The model under review builds one solid part; all positions refer to its coordinate system, in mm. A direction names the side the tool comes from. Round coordinates to 2 decimals unless told otherwise and drop trailing zeros. Order: outer loops, then holes, each group sorted by start corner. A loop starts at its lowest first (then second) coordinate and runs counter-clockwise, first axis right, second up. Notation, with made-up numbers: M 20,-13 L 30,-13 A16 cw 30,-9 Z; hole C 58.25,-1.75 d5. An arc over 180 degrees is marked long. Answer as a JSON object with one key per item and string values. Group by question number.
1) The part is to be moulded in two halves that separate along X. For faces 1 (the flat face through (-17, 16, -24)), 2 (the conical face through (-9.1, 9, 18.8)), 3 (the flat face through (-24, 0, 0)), say which applies: +X half, -X half, draft (parallel to the pull), parting line (faces both ways), or undercut.
2) For faces 4 (the flat face through (-17, 16, 24)), 5 (the conical face through (9.1, -9, 18.8)), list the 3-axis set-ups (+Z, -Z, +X, -X, +Y, -Y) from which the entire face can be reached by the end or side of a thin tool; tool diameter is ignored.
3) To check wall thickness, follow line 1 (X direction, y = 0, z = 4.5); line 2 (Y direction, x = -0.5, z = 5.5); line 3 (X direction, y = -2, z = 8). State the ranges of each line that lie inside material, in increasing order.
4) Insertion check: pin 1 Ø6 at (x, y) = (-17, 0) entering from +Z. The pin has a flat end and moves straight along its axis. Give the tip position at first contact, or say it passes through.
5) Consider section B-B, the plane x = -17. Write out the cut boundary in (y, z), then the cut area to 3 significant figures.
6) Consider section A-A, the plane z = -10. Write out the cut boundary in (x, y), then the cut area to 3 significant figures.
```python
from build123d import *

# Parameters (mm, degrees)
F0_W           = 48
F0_H           = 48
F1_DEPTH       = 24
F2_R           = 9
F3_DEPTH       = 48
F6_D           = 18
F6_CSINK_D     = 36
F6_CSINK_ANGLE = 90
F4_R           = 9
F7_DEPTH       = 48


with BuildPart() as f1:
    # F0 (on Front) → F1 (new body, symmetric)
    with BuildSketch(Plane.XZ):
        Rectangle(F0_W, F0_H)
    extrude(amount=F1_DEPTH, both=True)

    # F2 (on face) → F3 (cut)
    with BuildSketch(Plane.XZ.offset(24)):
        with Locations((0, 24)):
            Circle(F2_R)
        with Locations((0, -24)):
            Circle(F2_R)
    extrude(amount=-F3_DEPTH, mode=Mode.SUBTRACT)

    # F6 (through all)
    with Locations(Plane.XY.offset(24)):
        with Locations((0, 0)):
            CounterSinkHole(F6_D / 2, F6_CSINK_D / 2, counter_sink_angle=F6_CSINK_ANGLE)

    # F4 (on face) → F7 (cut)
    with BuildSketch(Plane.YZ.offset(24)):
        with Locations((0, 24)):
            Circle(F4_R)
        with Locations((0, -24)):
            Circle(F4_R)
    extrude(amount=-F7_DEPTH, mode=Mode.SUBTRACT)


solid = f1.part
```
Results list:
{
 "1": {"face 1": "draft", "face 2": "undercut", "face 3": "-X half"},
 "2": {"face 4": "+Z, +X, -X, +Y, -Y", "face 5": "+Z"},
 "3": {"line 1": "-24 to -9, 9 to 24", "line 2": "-24 to -8.99, 8.99 to 24", "line 3": "-24 to -8.77, 8.77 to 24"},
 "4": {"pin 1": "z = 15.51"},
 "5": {"outline": "M -24,-24 L -9,-24 A9 cw 9,-24 L 24,-24 L 24,24 L 9,24 A9 cw -9,24 L -24,24 Z", "area": "2,050 mm^2"},
 "6": {"outline": "M -24,-24 L 24,-24 L 24,24 L -24,24 Z; hole C 0,0 d18", "area": "2,050 mm^2"}
}
